```python
from build123d import *

# Parameters (mm, degrees)
EXTRUDE_THIN1_DEPTH = 381
FILLET1_R           = 1.27


with BuildPart() as part:
    # Sketch1 → Extrude-Thin1 (new body)
    with BuildSketch(Plane.XY):
        with BuildLine():
            Line((0, 0), (-3.96875, 0))
            Line((-3.96875, 0), (-3.96875, 5.55625))
            Line((-3.96875, 5.55625), (-7.9375, 5.55625))
            ThreePointArc((-7.9375, 5.55625), (-5.405853735, 15.931849892), (-10.986883491, 25.037585051))
            Line((-10.986883491, 25.037585051), (-15.820176145, 28.534612317))
            ThreePointArc((-15.820176145, 28.534612317), (-17.269464928, 32.972682848), (-13.49375, 35.71875))
            Line((-13.49375, 35.71875), (-13.49375, 38.1))
            Line((-13.49375, 38.1), (0, 38.1))
            Line((0, 38.1), (0, 36.83))
            Line((0, 36.83), (-12.22375, 36.83))
            Line((-12.22375, 36.83), (-12.22375, 34.13125))
            ThreePointArc((-12.22375, 34.13125), (-15.782927412, 33.179306943), (-15.075719779, 29.563536375))
            Line((-15.075719779, 29.563536375), (-10.242427125, 26.06650911))
            ThreePointArc((-10.242427125, 26.06650911), (-4.381358563, 17.296641703), (-5.659480864, 6.82625))
            Line((-5.659480864, 6.82625), (-2.69875, 6.82625))
            Line((-2.69875, 6.82625), (-2.69875, 1.27))
            Line((-2.69875, 1.27), (0, 1.27))
            Line((0, 1.27), (0, 0))
        make_face()
    extrude(amount=-EXTRUDE_THIN1_DEPTH)

    # Fillet1
    fillet1_edges = [part.edges().sort_by_distance(p)[0] for p in [
        (-3.96875, 0, -190.5),
        (-7.9375, 5.55625, -190.5),
        (-13.49375, 38.1, -190.5),
        (-12.22375, 34.13125, -190.5),
        (-2.69875, 6.82625, -190.5),
    ]]
    fillet(fillet1_edges, radius=FILLET1_R)


solid = part.part
```
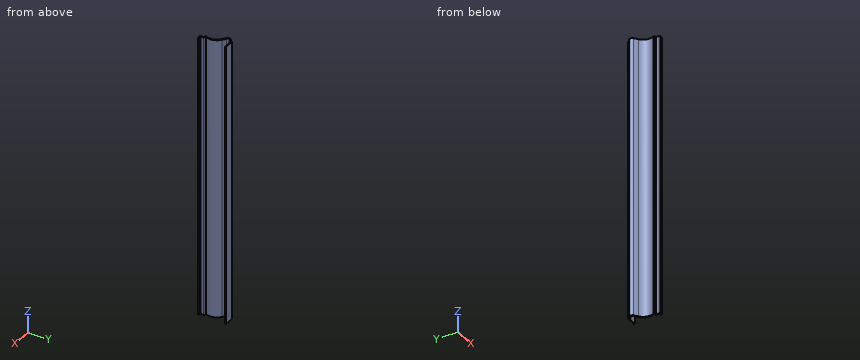
Part model, mm, in its own coordinate system. Coordinates: 2 decimals unless noted, no trailing zeros. Order: outer loops, then holes, each group sorted by start corner. A loop starts at its lowest first (then second) coordinate and runs counter-clockwise, first axis right, second up. Notation, with made-up numbers: (29.5, 38.25) - (63.5, 38.25) arc R29 ccw to (63.5, 74.25) - close; hole circle Ø4 at (-35.5, 87). An arc over 180 degrees is marked (long way). Return JSON: item names as keys, results as strings. Group by question number.
Item 1: Cut at B-B (y = 15.5). List the corners of the cut face in (x, z).
Item 2: Pin check, flat tips, straight feed: pin 1 (0.5 mm diameter, centred on x = -4.5, z = -140.5, fed in from -Y); pin 2 (6 mm diameter, centred on x = -15.5, z = -132, fed in from +Y); pin 3 (4.5 mm diameter, centred on y = 4.5, z = -167.5, fed in from +X). Stop position of each tip, or through.
Item 3: Cut at A-A (z = -106.5). List the corners of the cut face in (x, y), plus the area to 3 significant figures.
Item 4: Drill centre lines: probe 1 along Y at (x, z) = (-9.75, -16); probe 2 along X at (y, z) = (14, -164.5); probe 3 along Y at (x, z) = (-11.5, -334.5). Where is each one in solid material? Low to high. Write a range as from..to.
Check values:
{
 "1": {"outline": "(-5.35, -381) - (-4.07, -381) - (-4.07, 0) - (-5.35, 0) - close"},
 "2": {"pin 1": "stops at y = 5.56", "pin 2": "stops at y = 38.07", "pin 3": "stops at x = -2.7"},
 "3": {"outline": "(-15.82, 28.53) - (-10.99, 25.04) arc R13.89 cw to (-6.79, 7.41) arc R1.27 ccw to (-5.66, 5.56) - (-3.97, 5.56) - (-3.97, 1.27) arc R1.27 ccw to (-2.7, 0) - (0, 0) - (0, 1.27) - (-2.7, 1.27) - (-2.7, 5.56) arc R1.27 ccw to (-3.97, 6.83) - (-5.66, 6.83) arc R15.16 ccw to (-10.24, 26.07) - (-15.08, 29.56) arc R2.7 cw to (-13.49, 34.45) arc R1.27 ccw to (-12.22, 35.72) - (-12.22, 36.83) - (0, 36.83) - (0, 38.1) - (-12.22, 38.1) arc R1.27 ccw to (-13.49, 36.83) - (-13.49, 35.72) arc R3.97 ccw to start", "area": "79.1 mm2"},
 "4": {"probe 1": "y = 24.03..25.69, 36.83..38.1", "probe 2": "x = -5.24..-3.97", "probe 3": "y = 25.41..26.98, 36.83..38.1"}
}
